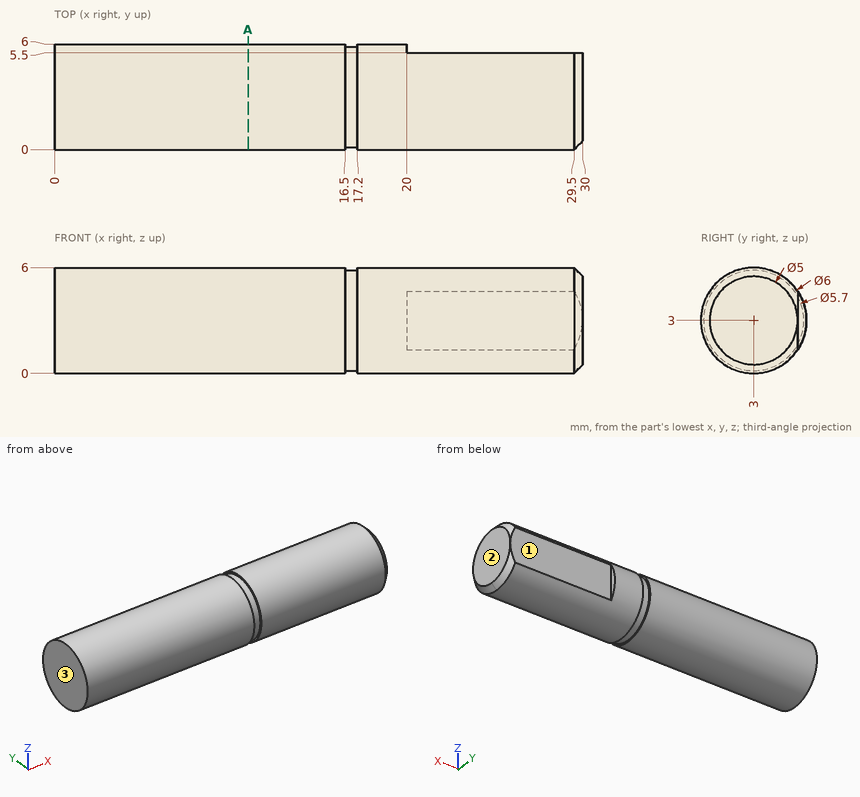
Geometry: see drawing. Coordinates: mm, zero at the bounding-box minimum. Coordinates: 2 decimals unless noted, no trailing zeros. Order: outer loops, then holes, each group sorted by start corner. A loop starts at its lowest first (then second) coordinate and runs counter-clockwise, first axis right, second up. Notation, with made-up numbers: (-40, 40) - (-10, 40) arc R16 cw to (-10, 52) - close; hole circle Ø1 at (44.5, -37). An arc over 180 degrees is marked (long way). Return JSON: item names as keys, results as strings.
Q1. First-contact query: pin 1 (1.5 mm diameter, centred on x = 15.5, y = 2, fed in from +Z); pin 2 (1 mm diameter, centred on x = 4, y = 4.5, fed in from -Z); pin 3 (3.5 mm diameter, centred on x = 25.5, z = 2.5, fed in from +Y). Flat tips, straight axial feed; report the tip coordinate or a pass-through.
The answers:
{"pin 1": "stops at z = 5.99", "pin 2": "stops at z = 0.17", "pin 3": "stops at y = 5.5"}
Q2. Draft query along X for the marked faces 1, 2 and 3. Return one class per face: +X half, -X half, draft (parallel to the pull), parting line (faces both ways), or undercut.
The answers:
{"face 1": "draft", "face 2": "+X half", "face 3": "-X half"}
Q3. Cut plane A-A (x = 11). Return loops of the section in (y, z).
The answers:
{"outline": "circle Ø6 at (3, 3)"}
Q4. Ray query, probe 1 along Z at (x, y) = (5, 3.1); probe 2 along Z at (x, y) = (22.5, 1.65); probe 3 along X at (y, z) = (4.55, 5.15). Return the intervals inside material, ascending.
The answers:
{"probe 1": "z = 0 to 6", "probe 2": "z = 0.32 to 5.68", "probe 3": "x = 0 to 29.85"}
